Autodesk Inventor part; units mm, degrees
ref_plane "Work Plane1" through (-0.5334, -0.3048, 5.08) normal (-1, 0, 0) x (0, 0, 1)
ref_plane "YZ Plane" through (0, 0, 0) normal (1, 0, 0) x (0, 1, 0)
ref_plane "XZ Plane" through (0, 0, 0) normal (0, 1, 0) x (-1, 0, 0)
sketch "Sketch1" plane through (0, 0, 0) normal (0, 0, 1) x (1, 0, 0)
  line L0 (0, 0) -> (12.6492, 0)
  line L1 (12.6492, 0) -> (12.6492, 11.176)
  line L2 (12.6492, 11.176) -> (0, 11.176)
  line L3 (0, 11.176) -> (0, 0)
  dimension "d0" = 12.6492
  dimension "d1" = 11.176
extrude "Extrusion1" add sketch "Sketch1" along normal blind 3.9624
sketch "Sketch2" plane through (0, 0, 0) normal (-1, 0, 0) x (0, 0, 1)
  line L0 (0, 0) -> (3.9624, 0)
  line L1 (3.9624, 11.176) -> (2.0574, 11.176)
  line L2 (2.0574, 11.176) -> (2.0574, 0)
  line L3 (2.0574, 0) -> (3.9624, 0)
  line L4 (3.9624, 0) -> (3.9624, 11.176)
  dimension "d4" = 1.905
ref_plane "Work Plane1" through (-0.5334, -0.3048, 5.08) normal (-1, 0, 0) x (0, 0, 1)
extrude "Extrusion2" add sketch "Sketch2" along normal up to surface (0.5334 mm away)
move faces "Move Face1" translate (0, 0.4064, 0) faces at (8.4328, 0, 2.0066)
move faces "Move Face2" translate (0, 0, 0.762) faces at (4.2164, 7.5861, 0)
properties part number "body_encoder"
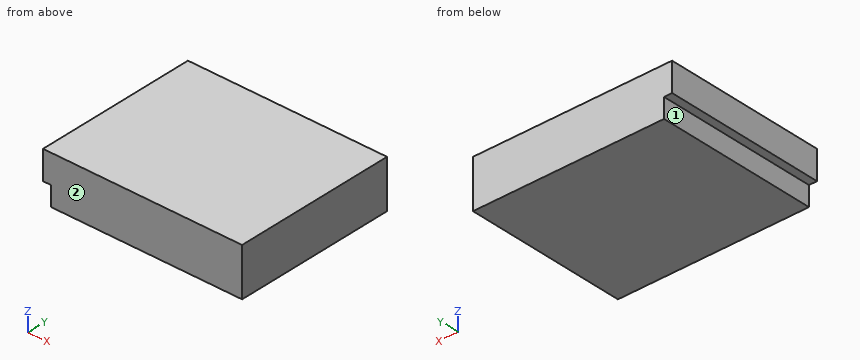
The listing builds one solid part. Answer for the finished solid, in the listing's coordinates (mm). Face numbers are marked on the shaded views. A direction names the side the tool comes from. Coordinates: 2 decimals unless noted, no trailing zeros. Loops run counter-clockwise (first coordinate to the right, second up) from the corner with the lowest first, then second, coordinate; pieces in that order, holes last. Notation, with made-up numbers: M 66,10.5 L 94,10.5 A10 ccw 94,15.5 Z; hole C 60.25,-32.75 d8. An arc over 180 degrees is marked long. Answer as CSV lines item,"result". Start each with the question number.
(1) The part is cut by section A-A (y = 7). Give the vertices of the cut face in (x, z).
(2) Given pin 1 (0.6 mm diameter, centred on y = 6, z = 1.5, fed in from -X), flat-ended and moving along its own axis, determine where the tip first touches the part or whether it passes through.
(3) For the marked faces 1 and 2, determine the directions among +Z, -Z, +X, -X, +Y, -Y from which every point of the face is accessible in a straight line to the end or side of a thin tool.
(4) The part is cut by section B-B (z = 1). Give the vertices of the cut face in (x, y), and give its area (3 significant figures).
(5) Find the intervals of material crossed by L1, parallel to X at y = 3.25, z = 1.45, in increasing order. Write a range as [from, to].
Determined:
1,outline,"M -0.53,2.06 L 0,2.06 L 0,0.76 L 12.65,0.76 L 12.65,3.96 L -0.53,3.96 Z"
2,pin 1,"x = 0"
3,face 1,"-Z, -X, +Y, -Y"
3,face 2,"+Z, -Z, +X, -X, -Y"
4,outline,"M 0,0.41 L 12.65,0.41 L 12.65,11.18 L 0,11.18 Z"
4,area,"136 mm2"
5,L1,"[0, 12.65]"
